Input: dimensioned drawing with shaded views. Units: mm. Origin: part minimum x, y, z. Coordinates: 2 decimals unless noted, no trailing zeros. Loops run counter-clockwise (first coordinate to the right, second up) from the corner with the lowest first, then second, coordinate; pieces in that order, holes last.
(1) Section D-D, the plane x = 77.5. Return loops of the section in (y, z).
(2) Section C-C, the plane x = 45.5. Return loops of the section in (y, z), then the cut area to 3 significant figures.
(3) Contact query for flat-ended pins moving along their axis: P1, Ø1, axis at x = 66.5, y = 4.5, coming from the +Z side; P2, Ø2.5, axis at x = 70.5, y = 2.5, coming from the -Z side; P3, Ø1, axis at y = 1, z = 13.5, coming from the +X side. Output: stop coordinate, or through.
(4) Section A-A, the plane z = 14. Return loops of the section in (x, y).
(5) Section B-B, the plane y = 3.35. Return loops of the section in (x, z), then the cut area to 3 significant figures.
(6) Line query: L1, parallel to X at y = 1.5, z = 1.75; L2, parallel to Z at x = 19, y = 0.25; L3, parallel to X at y = 1.6, z = 13. Output: solid intervals per line, ascending.
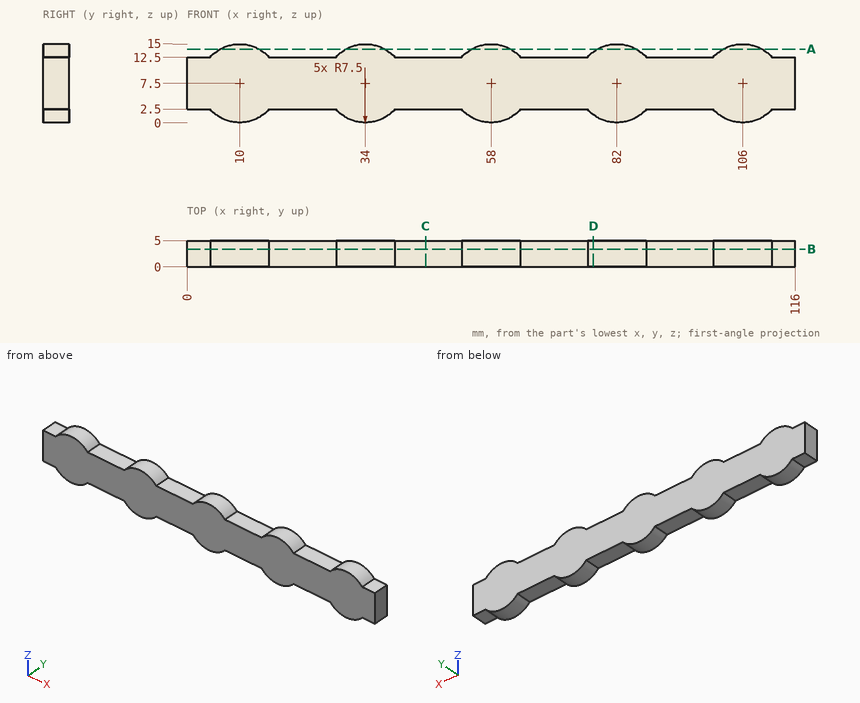
Report:
1. outline: (0, 1.5) - (5, 1.5) - (5, 13.5) - (0, 13.5) - close
2. outline: (0, 2.5) - (5, 2.5) - (5, 12.5) - (0, 12.5) - close
2. area: 50.0 mm2
3. P1: stops at z = 12.5
3. P2: stops at z = 2.5
3. P3: stops at x = 111.1
4. outline: (6.26, 0) - (13.74, 0) - (13.74, 5) - (6.26, 5) - close; (30.26, 0) - (37.74, 0) - (37.74, 5) - (30.26, 5) - close; (54.26, 0) - (61.74, 0) - (61.74, 5) - (54.26, 5) - close; (78.26, 0) - (85.74, 0) - (85.74, 5) - (78.26, 5) - close; (102.26, 0) - (109.74, 0) - (109.74, 5) - (102.26, 5) - close
5. outline: (0, 2.5) - (4.41, 2.5) arc R7.5 ccw to (15.59, 2.5) - (28.41, 2.5) arc R7.5 ccw to (39.59, 2.5) - (52.41, 2.5) arc R7.5 ccw to (63.59, 2.5) - (76.41, 2.5) arc R7.5 ccw to (87.59, 2.5) - (100.41, 2.5) arc R7.5 ccw to (111.59, 2.5) - (116, 2.5) - (116, 12.5) - (111.59, 12.5) arc R7.5 ccw to (100.41, 12.5) - (87.59, 12.5) arc R7.5 ccw to (76.41, 12.5) - (63.59, 12.5) arc R7.5 ccw to (52.41, 12.5) - (39.59, 12.5) arc R7.5 ccw to (28.41, 12.5) - (15.59, 12.5) arc R7.5 ccw to (4.41, 12.5) - (0, 12.5) - close
5. area: 1,350 mm2
6. L1: x = 5.18 to 14.82, 29.18 to 38.82, 53.18 to 62.82, 77.18 to 86.82, 101.18 to 110.82
6. L2: z = 2.5 to 12.5
6. L3: x = 4.9 to 15.1, 28.9 to 39.1, 52.9 to 63.1, 76.9 to 87.1, 100.9 to 111.1
